Here's how the part is built. I have some questions about the finished solid (model axes, mm). Coordinates: 2 decimals unless noted, no trailing zeros. Write each loop counter-clockwise with the first axis right and the second up, starting at its lowest first coordinate (ties: lowest second). Pieces come first, ordered by that corner, then holes.
(1) Imagine slicing it at C-C, the plane y = 40. List the corners of the cut face in (x, z) for me.
(2) For pin 1 Ø2.5 at (y, z) = (35.5, -30.5) entering from +X; pin 2 Ø5 at (x, z) = (-10, -27.5) entering from +Y; pin 3 Ø1.3 at (x, z) = (-1, -18) entering from +Y, each with a flat end and sliding along its axis, tell me the tip position at first contact or that it passes through.
(3) Imagine slicing it at D-D, the plane x = -4.5. List the corners of the cut face in (y, z) for me.
(4) Imagine slicing it at B-B, the plane x = -59. List the corners of the cut face in (y, z) for me.
(5) Please list where these lines run through material, in increasing order: probe 1 along Z at (x, y) = (-63.5, 20.5); probe 2 along X at (y, z) = (36, -23.5); probe 3 along Y at (x, z) = (-38, 1.5).
(6) Imagine slicing it at A-A, the plane z = -12.5. List the corners of the cut face in (x, y) for me.
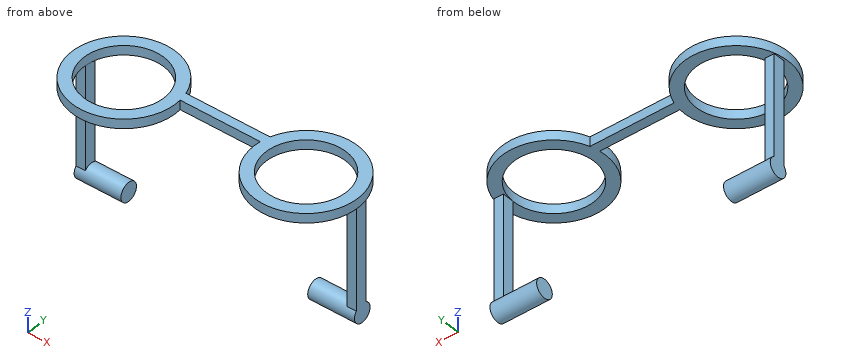
```python
from build123d import *

# Parameters (mm, degrees)
F0_R     = 10.795
F1_DEPTH = 2.54
F2_W     = 2.54
F2_H     = 3.175
F3_DEPTH = 27.94
F4_R     = 2.54
F5_DEPTH = 12.7
F6_R     = 2.54
F7_DEPTH = 12.7


with BuildPart() as f1:
    # F0 (on Top) → F1 (new body)
    with BuildSketch(Plane.XY):
        with BuildLine():
            Line((-25.97766, 37.288579), (-48.83766, 37.288579))
            ThreePointArc((-48.83766, 37.288579), (-75.791844, 30.04831), (-48.28081, 34.748579))
            Line((-48.28081, 34.748579), (-26.531821, 34.748579))
            ThreePointArc((-26.531821, 34.748579), (0.983912, 30.075824), (-25.97766, 37.288579))
        make_face()
        with Locations((-62.145926, 33.039937)):
            Circle(F0_R, mode=Mode.SUBTRACT)
        with Locations((-12.665021, 33.053661)):
            Circle(F0_R, mode=Mode.SUBTRACT)
    extrude(amount=F1_DEPTH)

    # F2 (on face) → F3 (join)
    with BuildSketch(Plane(origin=(0, 0, 0), x_dir=(1, 0, 0), z_dir=(0, 0, -1))):
        with Locations((-74.204193, -35.008655)):
            Rectangle(F2_W, F2_H)
        with Locations((-0.611128, -35.008655)):
            Rectangle(F2_W, F2_H)
    extrude(amount=F3_DEPTH)

    # F4 (on face) → F5 (join)
    with BuildSketch(Plane(origin=(-75.474193, 0, 0), x_dir=(0, -1, 0), z_dir=(-1, 0, 0))):
        with Locations((-35.361529, -29.579069)):
            Circle(F4_R)
    extrude(amount=-F5_DEPTH)

    # F6 (on face) → F7 (join)
    with BuildSketch(Plane.YZ.offset(0.658872)):
        with Locations((35.381455, -29.570073)):
            Circle(F6_R)
    extrude(amount=-F7_DEPTH)


solid = f1.part
```
Recorded:
1. outline: (-74.26, 0) - (-70.4, 0) - (-70.4, 2.54) - (-74.26, 2.54) - close; (-53.89, 0) - (-50.03, 0) - (-50.03, 2.54) - (-53.89, 2.54) - close; (-24.79, 0) - (-20.93, 0) - (-20.93, 2.54) - (-24.79, 2.54) - close; (-4.4, 0) - (-0.54, 0) - (-0.54, 2.54) - (-4.4, 2.54) - close
2. pin 1: stops at x = 0.66
2. pin 2: stops at y = 37.92
2. pin 3: stops at y = 36.6
3. outline: (21.72, 0) - (25.99, 0) - (25.99, 2.54) - (21.72, 2.54) - close; circle Ø5.08 at (35.38, -29.57); (40.12, 0) - (44.39, 0) - (44.39, 2.54) - (40.12, 2.54) - close
4. outline: (19.43, 0) - (22.71, 0) - (22.71, 2.54) - (19.43, 2.54) - close; (43.37, 0) - (46.65, 0) - (46.65, 2.54) - (43.37, 2.54) - close
5. probe 1: z = 0 to 2.54
5. probe 2: x = -75.47 to -72.93, -1.88 to 0.66
5. probe 3: y = 34.75 to 37.29
6. outline: (-75.47, 33.42) - (-72.93, 33.42) - (-72.93, 36.6) - (-75.47, 36.6) - close; (-1.88, 33.42) - (0.66, 33.42) - (0.66, 36.6) - (-1.88, 36.6) - close
